Work out the finished part from the listing and answer in its coordinate system (mm). Face numbers are marked on the shaded views. A direction names the side the tool comes from. Give positions to 0.01 mm unless a question says otherwise; leave off trailing zeros. Loops run counter-clockwise (first coordinate to the right, second up) from the corner with the lowest first, then second, coordinate; pieces in that order, holes last. Notation, with made-up numbers: (44.25, -34.5) - (52.25, -34.5) arc R29 cw to (52.25, -12.5) - close; hole circle Ø8 at (-36.75, 80). An arc over 180 degrees is marked (long way). Use one line per item in the form item = value. Start each with the question number.
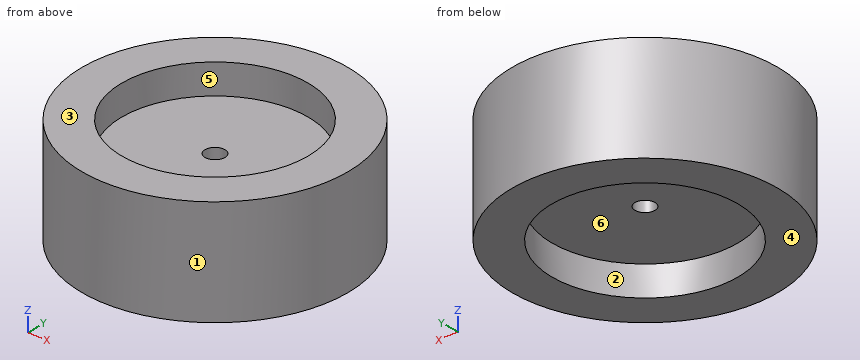
from build123d import *

# Parameters (mm, degrees)
F0_R     = 10
F1_DEPTH = 1.75
F2_R     = 0.75
F3_DEPTH = 10
F4_R     = 10
F4_R_2   = 7
F5_DEPTH = 4


with BuildPart() as f1:
    # F0 (on Top) → F1 (new body, symmetric)
    with BuildSketch(Plane.XY):
        Circle(F0_R)
    extrude(amount=F1_DEPTH, both=True)

    # F2 (on face) → F3 (cut, symmetric)
    with BuildSketch(Plane.XY.offset(1.75)):
        Circle(F2_R)
    extrude(amount=F3_DEPTH, both=True, mode=Mode.SUBTRACT)

    # F4 (on Top) → F5 (join, symmetric)
    with BuildSketch(Plane.XY):
        Circle(F4_R)
        Circle(F4_R_2, mode=Mode.SUBTRACT)
    extrude(amount=F5_DEPTH, both=True)


solid = f1.part
1) A cutting plane is placed at D-D (y = 3.5). Give the vertices of the cut face in (x, z).
2) A tool of negligible diameter and unlimited length cuts with its end or side. For the marked faces 4, 5 and 6, from which of +Z, -Z, +X, -X, +Y, -Y can it reach the whole face along a straight path? Write none if from no direction.
3) A cutting plane is placed at A-A (y = 0). Give the vertices of the cut face in (x, z).
4) Determine the mould class of the marked faces 1, 2 and 3 for opening direction X: released by +X, released by -X, zero draft, split by the parting line, or undercut.
5) Find the intervals of material crossed by probe 1 along Y at (x, z) = (0.25, -3); probe 2 along Y at (x, z) = (0, 0.35); probe 3 along Z at (x, y) = (1.75, 0.5), in increasing order.
6) A cutting plane is placed at C-C (z = 3). Give the vertices of the cut face in (x, y), plus the area to 3 significant figures.
7) Flat-ended cylindrical pins translate along their axes: pin 1 Ø8 at (x, y) = (2, -5.5) entering from +Z; pin 2 Ø1 at (y, z) = (7.5, -1) entering from +X; pin 3 Ø1.5 at (x, z) = (4, 1) entering from -Y; pin 4 Ø4 at (x, y) = (-0.5, -3) entering from -Z. Find the tip coordinate at first contact, or state that the pin passes through.
Answer sheet:
q1.outline = (-9.37, -4) - (-6.06, -4) - (-6.06, -1.75) - (6.06, -1.75) - (6.06, -4) - (9.37, -4) - (9.37, 4) - (6.06, 4) - (6.06, 1.75) - (-6.06, 1.75) - (-6.06, 4) - (-9.37, 4) - close
q2.face_4 = -Z, +X, -X, +Y, -Y
q2.face_5 = +Z
q2.face_6 = -Z
q3.outline = (-10, -4) - (-7, -4) - (-7, -1.75) - (-0.75, -1.75) - (-0.75, 1.75) - (-7, 1.75) - (-7, 4) - (-10, 4) - close; (0.75, -1.75) - (7, -1.75) - (7, -4) - (10, -4) - (10, 4) - (7, 4) - (7, 1.75) - (0.75, 1.75) - close
q4.face_1 = split by the parting line
q4.face_2 = undercut
q4.face_3 = zero draft
q5.probe_1 = -10 to -7, 7 to 10
q5.probe_2 = -10 to -0.75, 0.75 to 10
q5.probe_3 = -1.75 to 1.75
q6.outline = circle Ø20 at (0, 0); hole circle Ø14 at (0, 0)
q6.area = 160 mm²
q7.pin_1 = 4
q7.pin_2 = 7.14
q7.pin_3 = -9.46
q7.pin_4 = -1.75
